Autodesk Inventor part; units mm, degrees
ref_plane "Middle joining plane" through (0, -22.5, 0) normal (0, 1, 0) x (-1, 0, 0)
ref_plane "YZ Plane" through (0, 0, 0) normal (1, 0, 0) x (0, 1, 0)
ref_plane "XY Plane" through (0, 0, 0) normal (0, 0, 1) x (1, 0, 0)
sketch "Sketch1" plane through (0, 0, 0) normal (0, 0, 1) x (1, 0, 0)
  line L0 (-110, 22.5) -> (110, 22.5)
  line L1 (110, 22.5) -> (110, -22.5)
  line L2 (110, -22.5) -> (-110, -22.5)
  line L3 (-110, -22.5) -> (-110, 22.5)
  point P0 (0, 0)
  point P1 (110, 0)
  point P2 (0, 22.5)
  dimension "d0" = 220
  dimension "d1" = 45
extrude "Extrusion1" add sketch "Sketch1" along normal blind 15
sketch "Sketch2" plane through (0, 0, 15) normal (0, 0, 1) x (1, 0, 0)
  line L0 (-105, 15) -> (-55, 15) construction
  line L1 (-105, 12.5) -> (-55, 12.5)
  line L2 (-55, 17.5) -> (-105, 17.5)
  arc A0 (-105, 17.5) -> (-105, 12.5) centre (-105, 15) ccw
  arc A1 (-55, 12.5) -> (-55, 17.5) centre (-55, 15) ccw
  line L3 (-105, -15) -> (-55, -15) construction
  line L4 (-105, -17.5) -> (-55, -17.5)
  line L5 (-55, -12.5) -> (-105, -12.5)
  arc A2 (-105, -12.5) -> (-105, -17.5) centre (-105, -15) ccw
  arc A3 (-55, -17.5) -> (-55, -12.5) centre (-55, -15) ccw
  line L6 (-80, 15) -> (-80, -15) construction
  line L7 (-110, 22.5) -> (-110, -22.5)
  point P0 (0, 0)
  point P1 (-80, 0)
  dimension "d4" = 5
  dimension "d5" = 30
  dimension "d6" = 50
  dimension "d7" = 5
extrude "Extrusion2" cut sketch "Sketch2" against normal through all
mirror "Mirror1" about plane through (0, 0, 0) normal (1, 0, 0) of "Extrusion2"
fillet "Fillet1" [suppressed]
chamfer "Chamfer1" [suppressed]
sketch "Sketch3" plane through (0, 0, 15) normal (0, 0, -1) x (-1, 0, 0)
  line L0 (-20, -11.5) -> (20, -11.5) construction
  line L1 (-110, 22.5) -> (110, 22.5)
  line L2 (110, -22.5) -> (-110, -22.5)
  point P0 (0, 0)
  point P1 (0, -11.5)
  dimension "d14" = 40
  dimension "d28" = 11
hole "Hole1" at (20, -11.5, 15) at (-20, -11.5, 15) direction (0, 0, -1) diameter 6 end through all counterbore diameter 12 counterbore depth 5
ref_plane "Middle joining plane" through (0, -22.5, 0) normal (0, 1, 0) x (-1, 0, 0)
mirror "Double short side - join solid" about plane through (0, -22.5, 0) normal (0, 1, 0)
fillet "Double plate outer corners - R2" radius 2 4 edges at (110, -67.5, 7.5) (-110, -67.5, 7.5) (-110, 22.5, 7.5) (110, 22.5, 7.5)
chamfer "Double plate perimeter - 0.5 mm chamfer" distance 0.5 angle 45 12 edges at (109.4142, 21.9142, 15) (0, 22.5, 15) (-109.4142, 21.9142, 15) (-110, -22.5, 15) (0, -67.5, 15) (110, -22.5, 15) (109.4142, 21.9142, 0) (110, -22.5, 0) (0, -67.5, 0) (-110, -22.5, 0) (-109.4142, 21.9142, 0) (0, 22.5, 0)
equation "\"d28\" = bolts"
equation "\"bolts\" = 11"
properties part number "clamp-foot-double" material "Aluminum 6061"
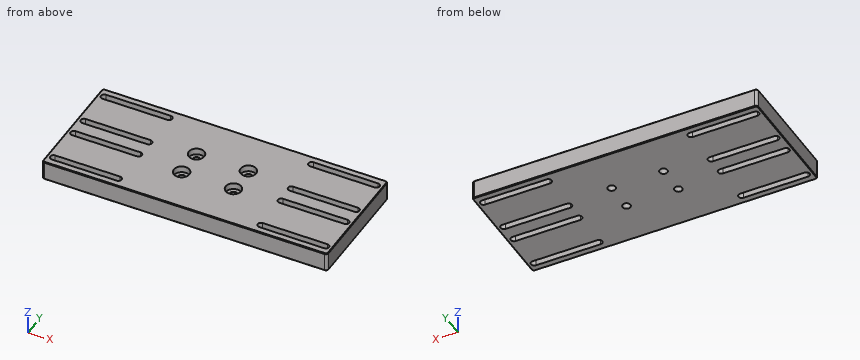
CAD build for the part. Positions are in the model's coordinates, mm. Coordinates: 2 decimals unless noted, no trailing zeros. Order: outer loops, then holes, each group sorted by start corner. A loop starts at its lowest first (then second) coordinate and runs counter-clockwise, first axis right, second up. Notation, with made-up numbers: M 65.5,20.5 L 100.5,20.5 A20 ccw 100.5,56.5 Z; hole C 64,36.5 d2. An arc over 180 degrees is marked long. Write each question's results on one line, items separated by ' | '. Start each with the question number.
Q1. Drill centre lines: probe 1 along Y at (x, z) = (64.5, 11.5); probe 2 along X at (y, z) = (-33.5, 12.35); probe 3 along X at (y, z) = (-11.5, 2.5). Where is each one in solid material? Low to high. Write a range as from..to.
Q2. Cut at B-B (z = 5). Count the separate pieces of the cut face and the enclosed holes in it, then the cut area to 3 significant figures.
Q3. Flat gauge pin, fed straight in: P1, Ø9.5, axis at x = -20, y = -33.5, coming from the +Z side. Where does the tip first touch, or does it go through?
Q4. Cut at A-A (x = 66). List the corners of the cut face in (y, z), then the cut area to 3 significant figures.
Found:
1) probe 1: -67.5..-62.5, -57.5..-32.5, -27.5..-17.5, -12.5..12.5, 17.5..22.5 | probe 2: -110..-26, -14..14, 26..110 | probe 3: -110..-23, -17..17, 23..110
2) separate pieces: 1 | enclosed holes: 12 | area: 17,500 mm²
3) P1: z = 10
4) outline: M -67.5,0.5 L -67,0 L -62.5,0 L -62.5,15 L -67,15 L -67.5,14.5 Z; M -57.5,0 L -32.5,0 L -32.5,15 L -57.5,15 Z; M -27.5,0 L -17.5,0 L -17.5,15 L -27.5,15 Z; M -12.5,0 L 12.5,0 L 12.5,15 L -12.5,15 Z; M 17.5,0 L 22,0 L 22.5,0.5 L 22.5,14.5 L 22,15 L 17.5,15 Z | area: 1,050 mm²
